from build123d import *

# Parameters (mm, degrees)
F1_DEPTH = 3
F2_SIZE  = 1.49999


# Not quite as in the source:
# - a fillet or chamfer is up to 0.001 mm smaller than in the source, because OpenCascade refuses the exact size


with BuildPart() as f1:
    # F0 (on Top) → F1 (new body)
    with BuildSketch(Plane.XY):
        Polygon((-50, 0), (0, 0), (9.9, 18.7), (34.4, 33.4), (61, 41.1), (28, 40.5), (-8, 28.8), align=None)
    extrude(amount=F1_DEPTH)

    # F2 (size 1.5 in the source; OpenCascade refuses exactly that, so slightly less here)
    f2_edges = [f1.edges().sort_by_distance(p)[0] for p in [
        (-29, 14.4, 3),
        (10, 34.65, 3),
        (10, 34.65, 0),
        (-29, 14.4, 0),
        (44.5, 40.8, 0),
        (44.5, 40.8, 3),
        (47.7, 37.25, 3),
        (47.7, 37.25, 0),
        (22.15, 26.05, 3),
        (22.15, 26.05, 0),
        (4.95, 9.35, 3),
        (4.95, 9.35, 0),
    ]]
    chamfer(f2_edges, length=F2_SIZE)


solid = f1.part
Verification items for the finished model (mm, model axes). Coordinates: 2 decimals unless noted, no trailing zeros. Order: outer loops, then holes, each group sorted by start corner. A loop starts at its lowest first (then second) coordinate and runs counter-clockwise, first axis right, second up. Notation, with made-up numbers: M 81.5,56.25 L 124.5,56.25 A26 cw 124.5,72.25 Z; hole C 50.5,59.25 d2. An arc over 180 degrees is marked long. Return JSON: item names as keys, results as strings.
1) Gauge pin test, flat end, axial feed: pin 1 (1 mm diameter, centred on y = 28, z = 2.5, fed in from -X). Record the tip position at first contact, or that the pin passes through.
Answer list:
{"pin 1": "x = -8.54"}
2) Thickness scan on L1, parallel to Y at x = -22, z = 1.9 (3 decimals); L2, parallel to Y at x = 20, z = 1.95; L3, parallel to X at y = 26, z = 0.6. Record the ranges inside material, lowest first. Write a range as [from, to].
Answer list:
{"L1": "[0, 18.715]", "L2": "[25.28, 37.43]", "L3": "[-10.49, 20.32]"}
3) Cross-section at C-C, the plane z = 2.05. Record the boundary of the cut face in (x, y), and give its area (3 significant figures).
Answer list:
{"outline": "M -49.03,0 L -0.62,0 L 9.49,19.09 L 34.18,33.91 L 56.86,40.47 L 28.09,39.95 L -7.75,28.3 Z", "area": "1,370 mm2"}
